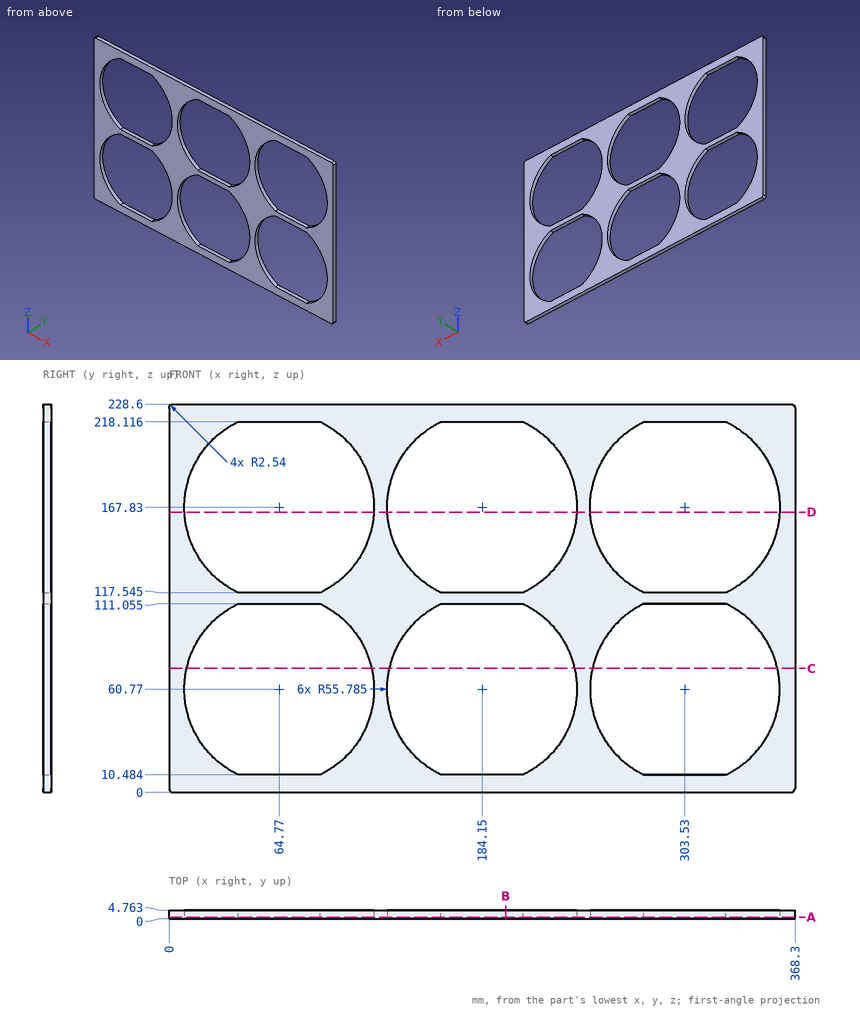
Input: dimensioned drawing with shaded views. Units: mm. Origin: part minimum x, y, z. Give positions to 0.01 mm unless a question says otherwise; leave off trailing zeros. Write each loop counter-clockwise with the first axis right and the second up, starting at its lowest first coordinate (ties: lowest second). Pieces come first, ordered by that corner, then holes. Notation, with made-up numbers: (14.25, 76) -> (54.25, 76) arc R27 ccw to (54.25, 107) -> close; hole circle Ø10 at (-36, 74.5). An arc over 180 degrees is marked (long way). Answer as a JSON object with one key per item and string values.
1. Cut plane D-D on z = 165. Output: boundary loops of the cut face in (x, y), and give its area (3 significant figures).
Ans:
{"outline": "(0, 0) -> (9.06, 0) -> (9.06, 4.76) -> (0, 4.76) -> close; (120.48, 0) -> (128.44, 0) -> (128.44, 4.76) -> (120.48, 4.76) -> close; (239.86, 0) -> (247.82, 0) -> (247.82, 4.76) -> (239.86, 4.76) -> close; (359.24, 0) -> (368.3, 0) -> (368.3, 4.76) -> (359.24, 4.76) -> close", "area": "162 mm^2"}
2. Cut plane B-B on x = 198. Output: boundary loops of the cut face in (y, z) (1 decimal), and give its area (3 significant figures).
Ans:
{"outline": "(0, 0) -> (4.8, 0) -> (4.8, 10.5) -> (0, 10.5) -> close; (0, 111.1) -> (4.8, 111.1) -> (4.8, 117.5) -> (0, 117.5) -> close; (0, 218.1) -> (4.8, 218.1) -> (4.8, 228.6) -> (0, 228.6) -> close", "area": "131 mm^2"}
3. Ray query, probe 1 along Z at (x, y) = (160, 3) (1 decimal); probe 2 along X at (y, z) = (0.9, 66); probe 3 along X at (y, z) = (1.55, 94) (1 decimal). Return the intervals inside material, ascending. Write a range as from..to.
Ans:
{"probe 1": "z = 0..10.5, 111.1..117.5, 218.1..228.6", "probe 2": "x = 0..9.23, 120.31..128.61, 239.69..247.99, 359.07..368.3", "probe 3": "x = 0..20, 109.6..139.3, 229..258.7, 348.3..368.3"}
4. Contact query for a flat-ended pin moving along its axis: pin 1 (1.4 mm diameter, centred on x = 298.5, y = 2.5, fed in from -Z). Output: stop coordinate, or through.
Ans:
{"pin 1": "stops at z = 0"}
5. Cut plane A-A on y = 0.9. Count the separate pieces of the cut face and the enclosed holes in it, and give its area (3 significant figures).
Ans:
{"separate pieces": "1", "enclosed holes": "6", "area": "27,700 mm^2"}
6. Cut plane C-C on z = 73. Output: boundary loops of the cut face in (x, y), and give its area (3 significant figures).
Ans:
{"outline": "(0, 0) -> (10.34, 0) -> (10.34, 4.76) -> (0, 4.76) -> close; (119.2, 0) -> (129.72, 0) -> (129.72, 4.76) -> (119.2, 4.76) -> close; (238.58, 0) -> (249.1, 0) -> (249.1, 4.76) -> (238.58, 4.76) -> close; (357.96, 0) -> (368.3, 0) -> (368.3, 4.76) -> (357.96, 4.76) -> close", "area": "199 mm^2"}
